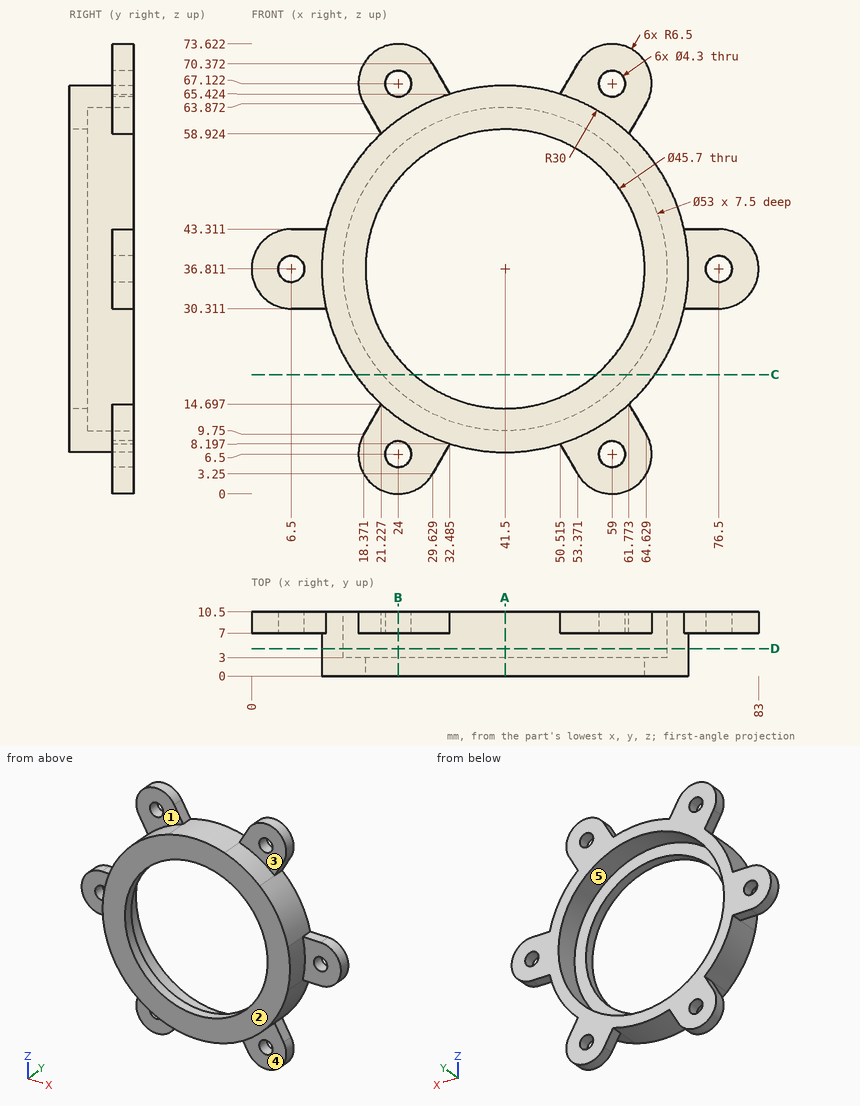
For this review, use the dimensioned drawing (mm, ordinates from the lowest corner) and the shaded views. A direction names the side the tool comes from. Give positions to 0.01 mm unless a question says otherwise; leave off trailing zeros. Order: outer loops, then holes, each group sorted by start corner. A loop starts at its lowest first (then second) coordinate and runs counter-clockwise, first axis right, second up.
1. Add section C-C, the plane z = 19.5. State the section outline as (x, y) points (1 decimal), then the cut area to 3 significant figures.
Solution:
outline: (17, 0) - (26.6, 0) - (26.6, 3) - (21.4, 3) - (21.4, 10.5) - (17, 10.5) - close; (56.4, 0) - (66, 0) - (66, 10.5) - (61.6, 10.5) - (61.6, 3) - (56.4, 3) - close
area: 124 mm2
2. To check wall thickness, follow L1, parallel to Z at x = 59, y = 9.8; L2, parallel to Z at x = 21, y = 7.5 (1 decimal); L3, parallel to Z at x = 41.5, y = 8.5. State the ranges of each line that lie inside material, in increasing order.
Solution:
L1: z = 0 to 4.35, 8.65 to 16.91, 56.71 to 64.97, 69.27 to 73.62
L2: z = 0.7 to 14.3, 14.9 to 20, 53.6 to 58.7, 59.3 to 72.9
L3: z = 6.81 to 10.31, 63.31 to 66.81
3. Add section D-D, the plane y = 4.5. State the section outline as (x, z) points (1 decimal).
Solution:
outline: circle Ø60 at (41.5, 36.8); hole circle Ø53 at (41.5, 36.8)
4. Add section A-A, the plane x = 41.5. State the section outline as (y, z) points.
Solution:
outline: (0, 6.81) - (10.5, 6.81) - (10.5, 10.31) - (3, 10.31) - (3, 13.96) - (0, 13.96) - close; (0, 59.66) - (3, 59.66) - (3, 63.31) - (10.5, 63.31) - (10.5, 66.81) - (0, 66.81) - close
5. Add section B-B, the plane x = 24. State the section outline as (y, z) points.
Solution:
outline: (0, 12.44) - (7, 12.44) - (7, 8.65) - (10.5, 8.65) - (10.5, 16.91) - (3, 16.91) - (3, 22.12) - (0, 22.12) - close; (0, 51.5) - (3, 51.5) - (3, 56.71) - (10.5, 56.71) - (10.5, 64.97) - (7, 64.97) - (7, 61.18) - (0, 61.18) - close; (7, 0) - (10.5, 0) - (10.5, 4.35) - (7, 4.35) - close; (7, 69.27) - (10.5, 69.27) - (10.5, 73.62) - (7, 73.62) - close
6. Mouldability with a two-part tool opening along X and no side actions: class the marked faces 4 and 5 as +X half, -X half, draft (parallel to the pull), parting line (faces both ways), or undercut.
Solution:
face 4: draft
face 5: undercut
7. For pin 1 Ø1.5 at (y, z) = (5, 33) entering from +X; pin 2 Ø4 at (y, z) = (2.5, 31.5) entering from -X; pin 3 Ø4.5 at (x, z) = (28.5, 5) entering from -Y; pin 4 Ø4 at (x, z) = (24, 67.12) entering from +Y (3 decimals), all flat-tipped, find the tip position at first contact; note any pin that passes through.
Solution:
pin 1: stops at x = 71.34
pin 2: stops at x = 11.68
pin 3: stops at y = 7
pin 4: passes through
8. Tool access review of the marked faces 1, 2 and 3: name each direction out of +Z, -Z, +X, -X, +Y, -Y from which nothing blocks a thin tool from reaching the whole face with its end or side.
Solution:
face 1: +Z, -X, -Y
face 2: +Z, -Z, +X, -X, -Y
face 3: +Z, +X, -Y
